Read the model definition and answer for the solid it produces. Units are mm, in the model's axes. Coordinates: 2 decimals unless noted, no trailing zeros. Order: outer loops, then holes, each group sorted by start corner. A loop starts at its lowest first (then second) coordinate and runs counter-clockwise, first axis right, second up. Notation, with made-up numbers: M 15.5,40 L 37.5,40 A20 ccw 37.5,59 Z; hole C 36.5,-19.75 d4. An arc over 180 degrees is marked long. Use a Markdown table: item, result. Add a question column.
1) Find section D-D on x = 0. Write down the section's boundary in (y, z).
2) Find section B-B on y = 1.8. Count the separate pieces of the cut face and the enclosed holes in it, plus the area to 3 significant figures.
3) Find the intervals of material crossed by probe 1 along X at (y, z) = (1.5, 46.5); probe 2 along X at (y, z) = (2.1, 0); probe 3 along Z at (x, y) = (-10, 2.5), in increasing order. Write a range as [from, to].
4) Find section A-A on z = 51. Write down the section's boundary in (x, y).
5) Each of these flat-tipped pins is pushed along its axis until it touches: pin 1 Ø1.5 at (y, z) = (3.5, 93.5) entering from +X; pin 2 Ø3 at (y, z) = (4.5, -12) entering from -X; pin 3 Ø2 at (x, z) = (46.5, -46.5) entering from +Y (3 decimals); pin 4 Ø1 at (y, z) = (4, 27) entering from -X. Where does it stop, or does it pass through?
6) Find section C-C on z = -38. Write down the section's boundary in (x, y).
from build123d import *

# Parameters (mm, degrees)
BOSS_EXTRU_1_DEPTH = 5
D_GAGEMENT_M31_D   = 3.4


with BuildPart() as part:
    # Esquisse1 → Boss.-Extru.1 (new body)
    with BuildSketch(Plane(origin=(0, 0, 0), x_dir=(1, 0, 0), z_dir=(0, 1, 0))):
        with BuildLine():
            Line((-15, -89.302855497), (-15, -105.302855497))
            ThreePointArc((-15, -105.302855497), (-13.828427125, -108.131282622), (-11, -109.302855497))
            Line((-11, -109.302855497), (11, -109.302855497))
            ThreePointArc((11, -109.302855497), (13.828427125, -108.131282622), (15, -105.302855497))
            Line((15, -105.302855497), (15, -89.302855497))
            ThreePointArc((15, -89.302855497), (19.455920451, -73.570722775), (31.5, -62.511998848))
            ThreePointArc((31.5, -62.511998848), (69.999576157, -0.243593621), (31.934306569, 62.291251905))
            ThreePointArc((31.934306569, 62.291251905), (26.226929885, 60.452488359), (28.065693431, 54.745111675))
            ThreePointArc((28.065693431, 54.745111675), (0, -61.52), (-28.065693431, 54.745111675))
            ThreePointArc((-28.065693431, 54.745111675), (-26.226929885, 60.452488359), (-31.934306569, 62.291251905))
            ThreePointArc((-31.934306569, 62.291251905), (-69.999576157, -0.243593621), (-31.5, -62.511998848))
            ThreePointArc((-31.5, -62.511998848), (-19.455920451, -73.570722775), (-15, -89.302855497))
        make_face()
    extrude(amount=BOSS_EXTRU_1_DEPTH)

    # Dégagement M31 (through all)
    with Locations(Plane(origin=(0, 5, 0), x_dir=(1, 0, 0), z_dir=(0, 1, 0))):
        with Locations((46.5, 46.5), (46.5, -46.5), (-46.5, -46.5), (-46.5, 46.5), (-10, -84.302855497), (10, -84.302855497), (10, -104.302855497), (-10, -104.302855497)):
            Hole(D_GAGEMENT_M31_D / 2)


solid = part.part
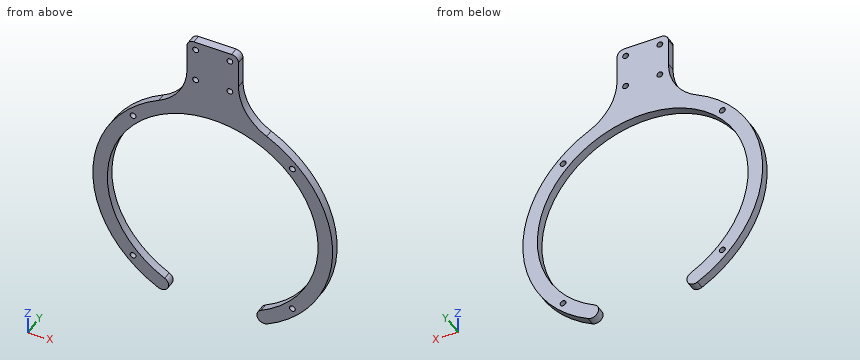
Check result:
| question | item | result |
|---|---|---|
| 1 | outline | M 0,61.52 L 5,61.52 L 5,109.3 L 0,109.3 Z |
| 2 | separate pieces | 1 |
| 2 | enclosed holes | 8 |
| 2 | area | 4,290 mm2 |
| 3 | probe 1 | x = [-52.32, -48.2], [-44.8, -40.28], [40.28, 44.8], [48.2, 52.32] |
| 3 | probe 2 | x = [-70, -61.52], [61.52, 70] |
| 3 | probe 3 | z = [60.7, 82.6], [86, 102.6], [106, 109.3] |
| 4 | outline | M -47.95,0 L -34.41,0 L -34.41,5 L -47.95,5 Z; M 34.41,0 L 47.95,0 L 47.95,5 L 34.41,5 Z |
| 5 | pin 1 | stops at x = 15 |
| 5 | pin 2 | stops at x = -69.21 |
| 5 | pin 3 | passes through |
| 5 | pin 4 | stops at x = -64.79 |
| 6 | outline | M -58.79,0 L -48.38,0 L -48.38,5 L -58.79,5 Z; M 48.38,0 L 58.79,0 L 58.79,5 L 48.38,5 Z |
